Check sheet for the modelled part. Datum: model origin and axes. Units: mm. Round coordinates to 2 decimals unless told otherwise and drop trailing zeros. Write each loop counter-clockwise with the first axis right and the second up, starting at its lowest first coordinate (ties: lowest second). Pieces come first, ordered by that corner, then holes. Notation, with made-up numbers: M 16.5,40.25 L 66.5,40.25 A12 ccw 66.5,44.25 Z; hole C 31,-9 d5. An arc over 180 degrees is marked long. One line per item, written item: value.
Autodesk Inventor part; units mm, degrees
ref_plane "YZ Plane" through (0, 0, 0) normal (1, 0, 0) x (0, 1, 0)
ref_plane "XZ Plane" through (0, 0, 0) normal (0, 1, 0) x (-1, 0, 0)
ref_plane "XY Plane" through (0, 0, 0) normal (0, 0, 1) x (1, 0, 0)
sketch "Sketch1" plane through (0, 0, 0) normal (1, 0, 0) x (0, 1, 0)
  line L0 (42.6763, 41.7539) -> (-33.5237, 41.7539)
  line L1 (-33.5237, 41.7539) -> (-33.5237, -85.2461)
  line L2 (-33.5237, -85.2461) -> (42.6763, -85.2461)
  line L3 (42.6763, -85.2461) -> (42.6763, 41.7539)
  point P0 (0, 0)
  dimension "d0" = 76.2
  dimension "d1" = 127
extrude "Extrusion1" add sketch "Sketch1" along normal blind 6.35
sketch "Sketch3" plane through (6.35, 0, 0) normal (1, 0, 0) x (0, 0, -1)
  arc A0 (59.8461, 10.9263) -> (59.8461, 23.6263) centre (59.8461, 17.2763) ccw
  arc A1 (21.7461, 23.6263) -> (21.7461, 10.9263) centre (21.7461, 17.2763) ccw
  line L0 (21.7461, 23.6263) -> (59.8461, 23.6263)
  line L1 (59.8461, 10.9263) -> (21.7461, 10.9263)
  line L2 (-41.7539, 42.6763) -> (-41.7539, -33.5237)
  line L3 (85.2461, 42.6763) -> (-41.7539, 42.6763)
  point P0 (0, 0)
  dimension "d4" = 38.1
  dimension "d5" = 101.6
  dimension "d6" = 25.4
  dimension "d7" = 25.4
  dimension "d9" = 6.35
extrude "Extrusion2" cut sketch "Sketch3" against normal blind 6.35
sketch "Sketch4" plane through (6.35, 0, 0) normal (1, 0, 0) x (0, 0, -1)
  circle A0 centre (-10.0039, -8.1237) radius 6.35
  line L0 (-41.7539, 42.6763) -> (-41.7539, -33.5237)
  line L1 (85.2461, 42.6763) -> (-41.7539, 42.6763)
  point P0 (0, 0)
  dimension "d12" = 31.75
  dimension "d13" = 50.8
  dimension "d14" = 12.7
extrude "Extrusion3" cut sketch "Sketch4" against normal blind 6.35
equation "\"d1\" = 1.66667 * d0"
equation "\"d2\" = 0.05 * d1"
equation "\"d4\" = 0.5 * d0"
equation "\"d5\" = 0.8 * d1"
equation "\"d6\" = 0.333333 * d0"
equation "\"d7\" = 0.333333 * d0"
equation "\"d9\" = d2"
equation "\"d10\" = 0.05 * d1"
equation "\"d12\" = 0.25 * d1"
equation "\"d13\" = 0.666667 * d0"
equation "\"d15\" = 0.05 * d1"
properties part number "8.2"
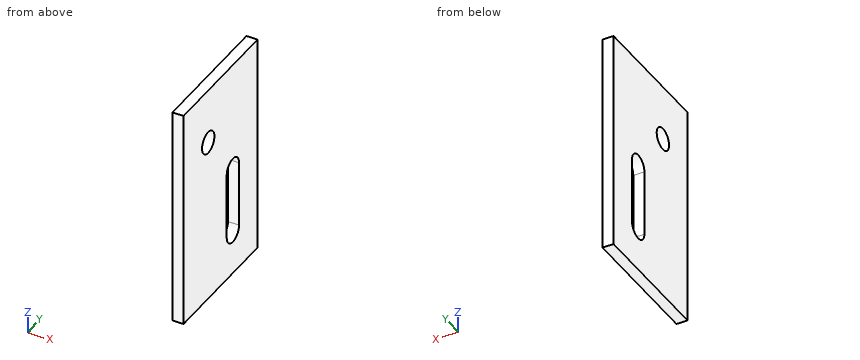
Q1. Sectioned sample at A-A on z = -44.5. Enter the section's corners in (x, y), and give its area (3 significant figures).
Completed:
outline: M 0,-33.52 L 6.35,-33.52 L 6.35,10.93 L 0,10.93 Z; M 0,23.63 L 6.35,23.63 L 6.35,42.68 L 0,42.68 Z
area: 403 mm^2
Q2. Sectioned sample at C-C on x = 1. Enter the section's corners in (y, z), and give its area (3 significant figures).
Completed:
outline: M -33.52,-85.25 L 42.68,-85.25 L 42.68,41.75 L -33.52,41.75 Z; hole C -8.12,10 d12.7; hole M 10.93,-59.85 A6.35 ccw 23.63,-59.85 L 23.63,-21.75 A6.35 ccw 10.93,-21.75 Z
area: 8,940 mm^2
Q3. Sectioned sample at B-B on y = 13.5. Enter the section's corners in (x, z), and give its area (3 significant figures).
Completed:
outline: M 0,-85.25 L 6.35,-85.25 L 6.35,-64.95 L 0,-64.95 Z; M 0,-16.64 L 6.35,-16.64 L 6.35,41.75 L 0,41.75 Z
area: 500 mm^2
Q4. Scan lines: line 1 (Y direction, x = 2.25, z = -37.5); line 2 (Z direction, x = 3.5, y = 13.5); line 3 (Z direction, x = 4, y = 12.5). Record each from-to range of solid material in increasing order. Write a range as [from, to].
Completed:
line 1: [-33.52, 10.93], [23.63, 42.68]
line 2: [-85.25, -64.95], [-16.64, 41.75]
line 3: [-85.25, -64.03], [-17.56, 41.75]
